Read the model definition and answer for the solid it produces. Units are mm, in the model's axes. A direction names the side the tool comes from. Coordinates: 2 decimals unless noted, no trailing zeros. Loops run counter-clockwise (first coordinate to the right, second up) from the corner with the lowest first, then second, coordinate; pieces in that order, holes last.
Q1. Which of the six approach directions +Z, -Z, +X, -X, +Y, -Y give full straight-line access (tool end or side, diameter ignored) to faces 1 (the face through (10, -7.938, 175)), 2 (the face through (10, -9.525, 175))?
Q2. Straight lines are drawn through the part: line 1 (X direction, y = -9.15, z = 12.5); line 2 (X direction, y = 3.5, z = 325); line 3 (Y direction, x = 4, z = 177) (1 decimal). For each, find the intervals that lie inside material, in ascending order.
Q3. Flat-ended cylindrical pins translate along their axes: P1, Ø8, axis at x = 9, y = -7, coming from the +Z side; P2, Ø5, axis at x = 10.32, z = 12.5, coming from the +Y side; P3, Ø3, axis at x = 10.32, z = 343.1, coming from the -Y side; P4, Ø1.5, axis at y = -4.5, z = 38.5, coming from the +X side. Find the tip coordinate at first contact, or state that the pin passes through.
Q4. Section B-B (y = 6.25) is taken. Give the vertices of the cut face in (x, z).
from build123d import *

# Parameters (mm, degrees)
BOSS_EXTRUDE1_DEPTH = 355.6
SKETCH3_R           = 1.984375
CUT_EXTRUDE1_DEPTH  = 1.5875


with BuildPart() as part:
    # Sketch2 → Boss-Extrude1 (new body)
    with BuildSketch(Plane.XY):
        Polygon((0, -9.525), (0, 9.525), (1.5875, 9.525), (1.5875, -7.9375), (19.05, -7.9375), (19.05, -9.525), align=None)
    extrude(amount=BOSS_EXTRUDE1_DEPTH)

    # Sketch3 → Cut-Extrude1 (cut)
    with BuildSketch(Plane(origin=(0, -7.9375, 0), x_dir=(1, 0, 0), z_dir=(0, 1, 0))):
        with Locations((10.31875, -12.5)):
            Circle(SKETCH3_R)
        with Locations((10.31875, -343.1)):
            Circle(SKETCH3_R)
    extrude(amount=-CUT_EXTRUDE1_DEPTH, mode=Mode.SUBTRACT)


solid = part.part
Numbers:
1. face 1: +Z, -Z, +X, +Y
1. face 2: +Z, -Z, +X, -X, -Y
2. line 1: x = 0 to 8.33, 12.3 to 19.05
2. line 2: x = 0 to 1.59
2. line 3: y = -9.5 to -7.9
3. P1: stops at z = 355.6
3. P2: stops at y = -7.94
3. P3: passes through
3. P4: stops at x = 1.59
4. outline: (0, 0) - (1.59, 0) - (1.59, 355.6) - (0, 355.6) - close
